Autodesk Inventor part; units mm, degrees
ref_plane "YZ Plane" through (0, 0, 0) normal (1, 0, 0) x (0, 1, 0)
ref_plane "XZ Plane" through (0, 0, 0) normal (0, 1, 0) x (-1, 0, 0)
ref_plane "XY Plane" through (0, 0, 0) normal (0, 0, 1) x (1, 0, 0)
sketch "puzzle" plane through (0, 0, 0) normal (0, 1, 0) x (-1, 0, 0)
  line L0 (0, -115) -> (-15, -115)
  line L1 (-135, -115) -> (-125, -115)
  line L2 (-135, -115) -> (-150, -115)
  line L3 (-75, -115) -> (-65, -115)
  line L4 (-75, -115) -> (-85.0002, -115)
  line L5 (-105, -135) -> (-94.9796, -135)
  line L6 (-94.9796, -135) -> (-115, -135)
  line L7 (-65, -115) -> (-60, -115)
  line L8 (-60, -125) -> (-63, -125)
  arc A0 (-60, -125) -> (-60, -115) centre (-60, -120) ccw
  arc A1 (-63, -125) -> (-63, -135) centre (-63, -130) ccw
  line L9 (-85.0002, -115) -> (-90.0002, -115)
  line L10 (-94.9796, -135) -> (-89.9796, -135)
  arc A2 (-90.0002, -115) -> (-90, -125) centre (-90.0002, -120) ccw
  arc A3 (-89.9796, -135) -> (-90, -125) centre (-89.9796, -130) ccw
  line L11 (-115, -135) -> (-120, -135)
  line L12 (-125, -115) -> (-120, -115)
  arc A4 (-120, -125) -> (-120, -115) centre (-120, -120) ccw
  arc A5 (-120, -125) -> (-120, -135) centre (-120, -130) ccw
  line L13 (0, -115) -> (-30, -115)
  line L14 (-63, -135) -> (-32.98, -135)
  line L15 (-32.98, -135) -> (-32, -135)
  line L16 (-30, -115) -> (-32, -115)
  arc A6 (-32, -115) -> (-32, -125) centre (-32, -120) ccw
  arc A7 (-32, -135) -> (-32, -125) centre (-32, -130) ccw
  line L17 (0, -115) -> (0, -230)
  line L18 (0, -230) -> (-150, -230)
  line L19 (-150, -230) -> (-150, -115)
  point P0 (0, 0)
  dimension "d22" = 5
  dimension "d23" = 5
  dimension "d24" = 5
  dimension "d25" = 5
  dimension "d26" = 5
  dimension "d76" = 115
extrude "Extrusión4" add sketch "puzzle" along normal blind 5
sketch "Boceto4" plane through (0, 0, 0) normal (0, -1, 0) x (1, 0, 0)
  line L0 (0, -115) -> (0, -230)
  line L1 (32, -115) -> (0, -115)
  line L2 (0, -230) -> (10, -230)
  line L3 (150, -230) -> (0, -230)
  line L4 (10, -180) -> (0, -180)
  line L5 (0, -230) -> (0, -180)
  line L6 (10, -230) -> (50, -230)
  line L7 (50, -230) -> (50, -220)
  line L8 (50, -220) -> (10, -220)
  line L9 (10, -220) -> (10, -180)
  line L10 (150, -230) -> (100, -230)
  line L11 (100, -230) -> (100, -220)
  line L12 (100, -220) -> (140, -220)
  line L13 (140, -220) -> (140, -180)
  line L14 (140, -180) -> (150, -180)
  line L15 (150, -115) -> (150, -230)
  line L16 (150, -230) -> (150, -180)
  line L17 (70, -212.5) -> (80, -212.5)
  line L18 (80, -152.5) -> (70, -152.5)
  line L19 (45, -177.5) -> (45, -187.5)
  line L20 (105, -177.5) -> (105, -187.5)
  line L21 (83, -177.5) -> (83, -174.5)
  line L22 (83, -174.5) -> (80, -174.5)
  line L23 (80, -174.5) -> (80, -152.5)
  line L24 (83, -177.5) -> (105, -177.5)
  line L25 (80, -177.5) -> (80, -187.5)
  line L26 (80, -177.5) -> (70, -177.5)
  line L27 (67, -177.5) -> (67, -174.5)
  line L28 (67, -174.5) -> (70, -174.5)
  line L29 (67, -187.5) -> (67, -190.5)
  line L30 (67, -190.5) -> (70, -190.5)
  line L31 (67, -177.5) -> (45, -177.5)
  line L32 (67, -187.5) -> (45, -187.5)
  line L33 (70, -174.5) -> (70, -152.5)
  line L34 (70, -177.5) -> (70, -182.5)
  line L35 (70, -190.5) -> (70, -212.5)
  line L36 (80, -187.5) -> (70, -187.5)
  line L37 (70, -187.5) -> (70, -182.5)
  line L38 (80, -190.5) -> (83, -190.5)
  line L39 (83, -190.5) -> (83, -187.5)
  line L40 (80, -190.5) -> (80, -212.5)
  line L41 (83, -187.5) -> (105, -187.5)
  point P0 (0, 0)
extrude "Extrusión5" add sketch "Boceto4" along normal blind 25
sketch "Boceto5" plane through (0, 0, 0) normal (0, -1, 0) x (1, 0, 0)
  line L0 (85, -115) -> (68, -115)
  line L1 (68, -120) -> (85, -120)
  line L2 (68, -120) -> (68, -115)
  line L3 (85, -120) -> (85, -115)
  line L4 (32, -135) -> (63, -135)
  line L5 (47.5, -135) -> (38.5, -135)
  line L6 (38.5, -135) -> (56.5, -135)
  line L7 (56.5, -135) -> (56.5, -140)
  line L8 (56.5, -140) -> (38.5, -140)
  line L9 (38.5, -140) -> (38.5, -135)
  line L10 (120, -135) -> (89.9796, -135)
  line L11 (104.9898, -135) -> (94.9898, -135)
  line L12 (94.9898, -135) -> (104.9898, -135)
  line L13 (104.9898, -135) -> (114.9898, -135)
  line L14 (114.9898, -135) -> (114.9898, -140)
  line L15 (114.9898, -140) -> (94.9898, -140)
  line L16 (94.9898, -140) -> (94.9898, -135)
  point P0 (0, 0)
extrude "Extrusión6" add sketch "Boceto5" along normal blind 10
sketch "Boceto6" plane through (89.9796, 5, -135) normal (0, 0, 1) x (1, 0, 0)
  line L0 (10.0204, -5) -> (50.0204, -5)
  line L1 (25, -5) -> (15, -5)
  line L2 (25.0102, -5) -> (25.0102, -15)
  line L3 (25.0102, -5) -> (25.0102, -15)
  line L4 (25.0102, -15) -> (5.0102, -15)
  line L5 (25.0102, -15) -> (5.0102, -15)
  line L6 (15.0204, -5) -> (15.0204, -30)
  circle A0 centre (15.0204, -10) radius 1.6
  line L7 (-33.4796, -15) -> (-51.4796, -15)
  line L8 (-33.4796, -15) -> (-51.4796, -15)
  circle A1 centre (-42.4796, -10) radius 1.6
  point P0 (-89.9796, -5)
  dimension "d120" = 10
  dimension "d121" = 3.2
  dimension "d123" = 3.2
extrude "Extrusión7" cut sketch "Boceto6" against normal blind 10 contours A0 L6 | L6 A0 | A1
sketch "Boceto7" plane through (32, 5, -135) normal (0, 0, 1) x (1, 0, 0)
  circle A0 centre (15.5, -10) radius 1.6
  circle A1 centre (15.5, -10) radius 1.6
  point P0 (-32, -5)
extrude "Extrusión8" cut sketch "Boceto7" against normal blind 34
sketch "Boceto8" plane through (68, 0, -115) normal (0, 0, 1) x (1, 0, 0)
  line L0 (22.0002, 0) -> (-8, 0)
  line L1 (17, 0) -> (0, 0)
  line L2 (0, 0) -> (0, -10)
  line L3 (0, -10) -> (17, -10)
  line L4 (17, -10) -> (17, 0)
  circle A0 centre (8.5, -5) radius 1.6
  point P0 (-68, 0)
  dimension "d128" = 3.2
extrude "Extrusión9" cut sketch "Boceto8" against normal blind 5 contours A0
sketch "Boceto9" plane through (150, 0, -115) normal (1, 0, 0) x (0, 0, -1)
  line L0 (115, 5) -> (115, -25)
  line L1 (20, 0) -> (10, 0)
  line L2 (115, 0) -> (20, 0)
  line L3 (20, 0) -> (20, -25)
  line L4 (115, -25) -> (65, -25)
  line L5 (20, -25) -> (115, -25)
  line L6 (115, -25) -> (115, 0)
  line L7 (115, 5) -> (115, -25)
  point P0 (-115, 0)
sketch "Boceto10" plane through (140, 0, -180) normal (0, 0, 1) x (1, 0, 0)
  line L0 (0, 0) -> (0, -25)
  line L1 (10, 5) -> (10, -25)
  line L2 (0, 0) -> (10, 0)
  line L3 (10, 0) -> (10, -25)
  line L4 (10, -25) -> (0, -25)
  line L5 (0, -25) -> (0, 0)
  point P0 (-140, 0)
extrude "Extrusión10" add sketch "Boceto10" along normal blind 45
extrude "Extrusión11" add sketch "Boceto9" along normal blind 10
sketch "Boceto12" plane through (150, 0, -135) normal (0, 1, 0) x (1, 0, 0)
  line L0 (0, 0) -> (0, 95)
  line L1 (0, 0) -> (10, 0)
  line L2 (10, 0) -> (10, 95)
  line L3 (10, 95) -> (0, 95)
  line L4 (0, 95) -> (0, 0)
  point P0 (-150, -135)
extrude "Extrusión12" add sketch "Boceto12" along normal blind 4
properties part number "base auxiliar 2"
Work out the finished part from the listing and answer in its coordinate system (mm). A direction names the side the tool comes from. Give positions to 0.01 mm unless a question says otherwise; leave off trailing zeros. Order: outer loops, then holes, each group sorted by start corner. A loop starts at its lowest first (then second) coordinate and runs counter-clockwise, first axis right, second up.
1. For faces 1 (the flat face through (45, -12, -182)), 2 (the flat face through (100, -12, -225)), 3 (the flat face through (48, -1, -135)), determine the directions among +Z, -Z, +X, -X, +Y, -Y from which every point of the face is accessible in a straight line to the end or side of a thin tool.
Result sheet:
face 1: -Y
face 2: -Z, -Y
face 3: +Y, -Y
2. Section B-B, the plane y = -12.75 is taken. Give the number of separate pieces and of enclosed holes in the cut face, and give its area (3 significant figures).
Result sheet:
separate pieces: 3
enclosed holes: 1
area: 4,240 mm2
3. Straight lines are drawn through the part: L1, parallel to X at y = -5, z = -198.5; L2, parallel to Z at x = 72, y = -9.75; L3, parallel to X at y = -10.5, z = -159.5. For each, find the intervals that lie inside material, in ascending order.
Result sheet:
L1: x = 0 to 10, 70 to 80, 140 to 160
L2: z = -212.5 to -187.5, -177.5 to -152.5, -120 to -115
L3: x = 70 to 80, 140 to 160
4. The mould has two halves that part along Z. Classify faces 4 (the flat face through (150, 4.2, -147.7)), 5 (the flat face through (68, -12, -190.5)), 6 (the cylindrical face through (84.98, 2.46, -129.88)): released by +Z, released by -Z, zero draft, split by the parting line, or undercut.
Result sheet:
face 4: zero draft
face 5: released by -Z
face 6: undercut
5. Section D-D, the plane x = 47.5 is taken. Determine the outline of the cut face in (y, z).
Result sheet:
outline: (-25, -230) - (5, -230) - (5, -135) - (-3.4, -135) - (-3.4, -140) - (0, -140) - (0, -177.5) - (-25, -177.5) - (-25, -187.5) - (0, -187.5) - (0, -220) - (-25, -220) - close; (-10, -140) - (-6.6, -140) - (-6.6, -135) - (-10, -135) - close
6. Each of these flat-tipped pins is pushed along its axis until it touches: P1, Ø11, axis at x = 7, y = -10.5, coming from the +Z side; P2, Ø1.5, axis at x = 68, y = -8.5, coming from the -Z side; P3, Ø4, axis at y = -12.5, z = -143, coming from the -X side. Where does it stop, or does it pass through?
Result sheet:
P1: stops at z = -180
P2: stops at z = -190.5
P3: stops at x = 140
7. Section C-C, the plane z = -156.5 is taken. Determine the outline of the cut face in (x, y), and give its area (3 significant figures).
Result sheet:
outline: (0, 0) - (70, 0) - (70, -25) - (80, -25) - (80, 0) - (140, 0) - (140, -25) - (160, -25) - (160, 4) - (150, 4) - (150, 5) - (0, 5) - close
area: 1,540 mm2
8. Section A-A, the plane x = 76.5 is taken. Determine the outline of the cut face in (y, z).
Result sheet:
outline: (-25, -212.5) - (0, -212.5) - (0, -230) - (5, -230) - (5, -115) - (-3.4, -115) - (-3.4, -120) - (0, -120) - (0, -152.5) - (-25, -152.5) - (-25, -177.5) - (0, -177.5) - (0, -187.5) - (-25, -187.5) - close; (-10, -120) - (-6.6, -120) - (-6.6, -115) - (-10, -115) - close
